Verification items for the finished model (mm, model axes). A direction names the side the tool comes from. Give positions to 0.01 mm unless a question says otherwise; leave off trailing zeros. Write each loop counter-clockwise with the first axis right and the second up, starting at its lowest first coordinate (ties: lowest second). Pieces come first, ordered by that corner, then holes. Notation, with made-up numbers: M 53.5,21.5 L 62.5,21.5 A18 cw 62.5,48.5 Z; hole C -10.75,19.5 d9. An arc over 180 degrees is marked long. Write item = value, one per line.
from build123d import *

# Parameters (mm, degrees)
SKETCH_1_W               = 26
SKETCH_1_H               = 11.9
SKETCH_1_W_2             = 22
SKETCH_1_H_2             = 7.9
EXTRUDE_1_DEPTH          = 110
SKETCH_3_W               = 151.071145041
SKETCH_3_H               = 8.521608695
CUT_EXTRUDE_1_DEPTH      = 50
SKETCH_4_W               = 2.5
SKETCH_4_H               = 14.950427865
EXTRUDE_2_DEPTH          = 30
SKETCH_5_W               = 31
SKETCH_5_H               = 14.950427865
EXTRUDE_3_DEPTH          = 3
CUT_EXTRUDE_2_DEPTH      = 114.987971742
CUT_EXTRUDE_2_DEPTH_BACK = 10


with BuildPart() as part:
    # 草图1 → 凸台-拉伸1 (new body)
    with BuildSketch(Plane(origin=(0, 0, 0), x_dir=(0, 0, -1), z_dir=(1, 0, 0))):
        Rectangle(SKETCH_1_W, SKETCH_1_H)
        Rectangle(SKETCH_1_W_2, SKETCH_1_H_2, mode=Mode.SUBTRACT)
    extrude(amount=EXTRUDE_1_DEPTH)

    # 草图3 → 切除-拉伸1 (cut)
    with BuildSketch(Plane.XY.offset(13)):
        with Locations((72.322087123, 4.260804348)):
            Rectangle(SKETCH_3_W, SKETCH_3_H)
    extrude(amount=-CUT_EXTRUDE_1_DEPTH, mode=Mode.SUBTRACT)

    # 草图4 → 凸台-拉伸2 (add)
    with BuildSketch(Plane.ZY):
        with Locations((14.25, 1.525213933)):
            Rectangle(SKETCH_4_W, SKETCH_4_H)
        with Locations((-14.25, 1.525213933)):
            Rectangle(SKETCH_4_W, SKETCH_4_H)
    extrude(amount=-EXTRUDE_2_DEPTH)

    # 草图5 → 凸台-拉伸3 (add)
    with BuildSketch(Plane.ZY):
        with Locations((0, 1.525213933)):
            Rectangle(SKETCH_5_W, SKETCH_5_H)
    extrude(amount=EXTRUDE_3_DEPTH)

    # 草图6 → 切除-拉伸2 (cut, two sides: drawn at the far end of the back side and taken through both)
    with BuildSketch(Plane.XY.offset(-13).offset(-CUT_EXTRUDE_2_DEPTH_BACK)):
        with BuildLine():
            Line((18.563166245, 4.587279606), (12.192847179, 4.587279606))
            ThreePointArc((12.192847179, 4.587279606), (10.632355173, 2.837216293), (8.379481629, 2.187279606))
            Line((8.379481629, 2.187279606), (18.563166245, 2.187279606))
            ThreePointArc((18.563166245, 2.187279606), (19.763166245, 3.387279606), (18.563166245, 4.587279606))
        make_face()
        with BuildLine():
            Line((8.379481629, 4.587279606), (7.947587552, 4.587279606))
            Line((7.947587552, 4.587279606), (8.200962294, 4.460592236))
            ThreePointArc((8.200962294, 4.460592236), (8.854523462, 3.234366745), (7.912225197, 2.213168853))
            ThreePointArc((7.912225197, 2.213168853), (8.145495077, 2.193756878), (8.379481629, 2.187279606))
            ThreePointArc((8.379481629, 2.187279606), (10.632355173, 2.837216293), (12.192847179, 4.587279606))
            Line((12.192847179, 4.587279606), (8.379481629, 4.587279606))
        make_face()
        with BuildLine():
            Line((7.561289802, 4.780428481), (5.200962294, 5.960592236))
            ThreePointArc((5.200962294, 5.960592236), (4.689059665, 6.087024269), (4.172377695, 5.981814468))
            ThreePointArc((4.172377695, 5.981814468), (4.900896967, 4.01090385), (6.487977015, 2.633803302))
            ThreePointArc((6.487977015, 2.633803302), (6.700157723, 2.534954754), (6.917481998, 2.447995868))
            ThreePointArc((6.917481998, 2.447995868), (6.531358389, 3.782791625), (7.664305979, 4.587279606))
            Line((7.664305979, 4.587279606), (7.947587552, 4.587279606))
            Line((7.947587552, 4.587279606), (7.561289802, 4.780428481))
        make_face()
        with BuildLine():
            ThreePointArc((8.379481629, 4.587279606), (7.959141186, 4.636221447), (7.561289802, 4.780428481))
            Line((7.561289802, 4.780428481), (7.947587552, 4.587279606))
            Line((7.947587552, 4.587279606), (8.379481629, 4.587279606))
        make_face()
        with BuildLine():
            ThreePointArc((6.487977015, 2.633803302), (4.900896967, 4.01090385), (4.172377695, 5.981814468))
            ThreePointArc((4.172377695, 5.981814468), (3.464561317, 4.912033292), (4.127649665, 3.813966977))
            Line((4.127649665, 3.813966977), (6.487977015, 2.633803302))
        make_face()
        with BuildLine():
            Line((8.200962294, 4.460592236), (7.947587552, 4.587279606))
            Line((7.947587552, 4.587279606), (7.664305979, 4.587279606))
            ThreePointArc((7.664305979, 4.587279606), (6.531358389, 3.782791625), (6.917481998, 2.447995868))
            ThreePointArc((6.917481998, 2.447995868), (7.407734146, 2.300423879), (7.912225197, 2.213168853))
            ThreePointArc((7.912225197, 2.213168853), (8.854523462, 3.234366745), (8.200962294, 4.460592236))
        make_face()
    extrude(amount=CUT_EXTRUDE_2_DEPTH + CUT_EXTRUDE_2_DEPTH_BACK, mode=Mode.SUBTRACT)


solid = part.part
1) Tool access check on faces 1 (the flat face through (69, -3, -13)), 2 (the flat face through (15, 5, 13)), 3 (the flat face through (14, 4.587, 14)). Record the directions out of +Z, -Z, +X, -X, +Y, -Y that give a thin tool (end or side, any length) a straight path to the whole face; none if there is none.
From the geometry:
face_1 = -Z, +X, +Y, -Y
face_2 = +X, +Y
face_3 = +Z, -Z
2) Cross-section at B-B on y = -2.5. Record the boundary of the cut face in (x, z).
From the geometry:
outline = M -3,-15.5 L 30,-15.5 L 30,-13 L 110,-13 L 110,-11 L 0,-11 L 0,11 L 110,11 L 110,13 L 30,13 L 30,15.5 L -3,15.5 Z
3) Material ranges on probe 1 along Z at (x, y) = (3.5, -3.5); probe 2 along Z at (x, y) = (60, -3); probe 3 along X at (y, z) = (0.75, 1.5), recorded low to high. Write a range as from..to.
From the geometry:
probe_1 = -15.5..-11, 11..15.5
probe_2 = -13..-11, 11..13
probe_3 = -3..0
4) Cross-section at C-C on z = -2. Record the boundary of the cut face in (x, y).
From the geometry:
outline = M -3,-5.95 L 110,-5.95 L 110,-3.95 L 0,-3.95 L 0,9 L -3,9 Z
5) Cross-section at A-A on x = 89.5. Record the boundary of the cut face in (y, z).
From the geometry:
outline = M -5.95,-13 L 0,-13 L 0,-11 L -3.95,-11 L -3.95,11 L 0,11 L 0,13 L -5.95,13 Z
6) Draft check along X on faces 4 (the flat face through (30, 2, 14)), 5 (the flat face through (6.4, 5.36, 14.23)), 6 (the flat face through (5.291, 3.232, 14.233)), 7 (the flat face through (14, 1, -15.5)). Enter one of: +X half, -X half, draft (parallel to the pull), parting line (faces both ways), or undercut.
From the geometry:
face_4 = +X half
face_5 = undercut
face_6 = undercut
face_7 = draft
7) Depth check by flat-ended pin: P1, Ø1.8, axis at x = 78.5, y = -3.5, coming from the -Z side; P2, Ø2, axis at x = 68.5, y = -1.5, coming from the +Z side; P3, Ø1, axis at y = 1, z = -3.5, coming from the +X side. Enter the tip coordinate at first touch or a pass-through.
From the geometry:
P1 = -13
P2 = 13
P3 = 0
